The listing builds one solid part. Answer for the finished solid, in the listing's coordinates (mm). Face numbers are marked on the shaded views. A direction names the side the tool comes from. Give positions to 0.01 mm unless a question says otherwise; leave off trailing zeros. Write each loop counter-clockwise with the first axis right and the second up, starting at its lowest first coordinate (ties: lowest second). Pieces come first, ordered by that corner, then holes. Notation, with made-up numbers: M 32,18 L 59,18 A6 cw 59,26 Z; hole C -7,-34 d4. An arc over 180 degrees is marked long. Answer as a JSON object with one key per item and string values.
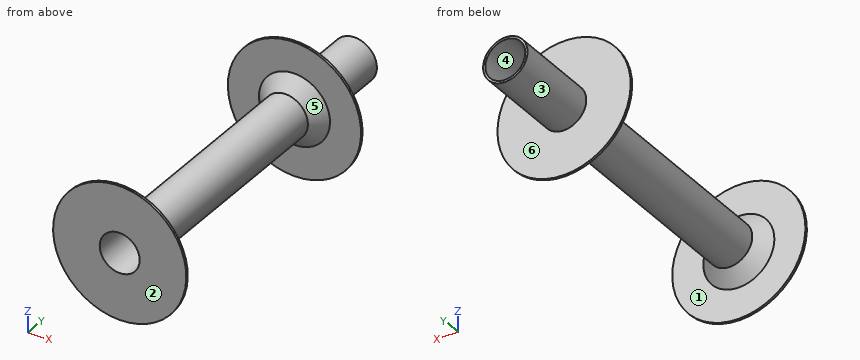
```python
from build123d import *

# Parameters (mm, degrees)
SKETCH1_R           = 50
BOSS_EXTRUDE1_DEPTH = 800
SKETCH3_R           = 45
CUT_EXTRUDE1_DEPTH  = 828.647267862


with BuildPart() as part:
    # Sketch1 → Boss-Extrude1 (new body)
    with BuildSketch(Plane(origin=(0, 0, 0), x_dir=(1, 0, 0), z_dir=(0, 1, 0))):
        with Locations(Location((0, 0, 0), (0, 0, 270))):
            Circle(SKETCH1_R)
    extrude(amount=BOSS_EXTRUDE1_DEPTH)

    # Sketch2 → Revolve1 (revolve)
    with BuildSketch(Plane.XY, mode=Mode.PRIVATE) as revolve1_sk:
        Polygon((0, 0), (150, 0), (150, 5), (80, 5), (0, 85), align=None)
        Polygon((0, 600), (150, 600), (150, 595), (80, 595), (0, 515), align=None)
    revolve(revolve1_sk.sketch.rotate(Axis((0, -31.169915786, 0), (0, 1, 0)), 90), axis=Axis((0, -31.169915786, 0), (0, 1, 0)))

    # Sketch3 → Cut-Extrude1 (cut, through all)
    with BuildSketch(Plane(origin=(0, 800, 0), x_dir=(1, 0, 0), z_dir=(0, 1, 0))):
        with Locations(Location((0, 0, 0), (0, 0, 270))):
            Circle(SKETCH3_R)
    extrude(amount=-CUT_EXTRUDE1_DEPTH, mode=Mode.SUBTRACT)


solid = part.part
```
1. The mould has two halves that part along Y. Classify the marked faces 4, 5 and 6: released by +Y, released by -Y, zero draft, split by the parting line, or undercut.
Verdict:
{"face 4": "zero draft", "face 5": "undercut", "face 6": "released by +Y"}
2. Consider line 1 along X through (y, z) = (446, 0); line 2 along Y through (x, z) = (-87.5, -6.5); line 3 along Y through (x, z) = (-59, 6). Determine where each line is inside the solid, lowest interval first.
Verdict:
{"line 1": "x = -50 to -45, 45 to 50", "line 2": "y = 0 to 5, 595 to 600", "line 3": "y = 0 to 25.7, 574.3 to 600"}
3. A cutting plane is placed at C-C, the plane y = 247.5. Give the vertices of the cut face in (x, z), plus the area to 3 significant figures.
Verdict:
{"outline": "C 0,0 d100; hole C 0,0 d90", "area": "1,490 mm2"}
4. A cutting plane is placed at A-A, the plane x = 0. Give the vertices of the cut face in (y, z), plus the area to 3 significant figures.
Verdict:
{"outline": "M 0,-150 L 5,-150 L 5,-80 L 35,-50 L 565,-50 L 595,-80 L 595,-150 L 600,-150 L 600,-50 L 800,-50 L 800,-45 L 0,-45 Z; M 0,45 L 800,45 L 800,50 L 600,50 L 600,150 L 595,150 L 595,80 L 565,50 L 35,50 L 5,80 L 5,150 L 0,150 Z", "area": "11,800 mm2"}
5. A cutting plane is placed at D-D, the plane z = -117. Give the vertices of the cut face in (x, y), plus the area to 3 significant figures.
Verdict:
{"outline": "M -93.87,0 L 93.87,0 L 93.87,5 L -93.87,5 Z; M -93.87,595 L 93.87,595 L 93.87,600 L -93.87,600 Z", "area": "1,880 mm2"}
6. For the marked faces 1, 2 and 3, determine the directions among +Z, -Z, +X, -X, +Y, -Y from which every point of the face is accessible in a straight line to the end or side of a thin tool.
Verdict:
{"face 1": "none", "face 2": "+Z, -Z, +X, -X, -Y", "face 3": "+Y"}
7. Flat-ended cylindrical pins translate along their axes: pin 1 (6 mm diameter, centred on x = 28, y = 637, fed in from +Z); pin 2 (8 mm diameter, centred on y = 589, z = 34.5, fed in from +X); pin 3 (6 mm diameter, centred on y = 603.5, z = 63, fed in from -X); pin 4 (2 mm diameter, centred on y = 249.5, z = 36.5, fed in from -X). Find the tip coordinate at first contact, or state that the pin passes through.
Verdict:
{"pin 1": "stops at z = 43.3", "pin 2": "stops at x = 70.35", "pin 3": "passes through", "pin 4": "stops at x = -35.21"}
8. A cutting plane is placed at B-B, the plane z = 0. Give the vertices of the cut face in (x, y), plus the area to 3 significant figures.
Verdict:
{"outline": "M -150,0 L -45,0 L -45,800 L -50,800 L -50,600 L -150,600 L -150,595 L -80,595 L -50,565 L -50,35 L -80,5 L -150,5 Z; M 45,0 L 150,0 L 150,5 L 80,5 L 50,35 L 50,565 L 80,595 L 150,595 L 150,600 L 50,600 L 50,800 L 45,800 Z", "area": "11,800 mm2"}
